Verification items for the finished model (mm, model axes). A direction names the side the tool comes from. Coordinates: 2 decimals unless noted, no trailing zeros. Loops run counter-clockwise (first coordinate to the right, second up) from the corner with the lowest first, then second, coordinate; pieces in that order, holes last. Notation, with made-up numbers: (3.5, -16) - (33.5, -16) arc R26 ccw to (33.5, 21) - close; hole circle Ø11 at (-1.5, 18). An arc over 180 degrees is marked (long way). One line per item, written item: value. Start each with the question number.
(1) Section check C-C (y = -56). Record the boundary of the cut face in (x, z), plus the area to 4 significant figures.
(2) Section check B-B (z = 581). Record the boundary of the cut face in (x, y).
(3) Section check A-A (x = 31). Record the boundary of the cut face in (y, z), plus the area to 3 significant figures.
(4) Gauge pin test, flat ends, axial feed: P1, Ø1, axis at y = -95, z = 428.5, coming from the -X side; P2, Ø0.9, axis at x = 1, z = 397, coming from the +Y side. Record the tip position at first contact, or that the pin passes through.
(5) Draft check along Y on faces 3 (the face through (2.9, -143, 320)), 4 (the face through (25, -149.5, 320)), 5 (the face through (0, -9, 320)), 6 (the face through (26, -152.4, 320)). Enter one of: +Y half, -Y half, draft (parallel to the pull), parting line (faces both ways), or undercut.
(6) Thickness scan on probe 1 along Y at (x, z) = (23.5, 321); probe 2 along X at (y, z) = (-13.5, 350.5); probe 3 along X at (y, z) = (-45, 486.5). Record the ranges inside material, lowest first. Write a range as [from, to].
(7) Set-up check for faces 1 (the face through (50.8, -75, 320)), 2 (the face through (2.9, -9, 320)): record each of +Z, -Z, +X, -X, +Y, -Y from which the full face is reachable in a straight line by a thin tool's end or side.
```python
from build123d import *

# Parameters (mm, degrees)
SALIENTE_EXTRUIR1_DEPTH = 650
REDONDEO1_R             = 2


with BuildPart() as part:
    # Croquis1 → Saliente-Extruir1 (new body)
    with BuildSketch(Plane.XY):
        Polygon((0, 0), (50.8, 0), (50.8, -152.4), (0, -152.4), (0, -137.4), (2.9, -137.4), (2.9, -149.5), (47.9, -149.5), (47.9, -2.9), (2.9, -2.9), (2.9, -15), (0, -15), align=None)
    extrude(amount=SALIENTE_EXTRUIR1_DEPTH)

    # Redondeo1
    redondeo1_edges = [part.edges().sort_by_distance(p)[0] for p in [
        (0, 0, 325),
        (50.8, 0, 325),
        (50.8, -152.4, 325),
        (0, -152.4, 325),
    ]]
    fillet(redondeo1_edges, radius=REDONDEO1_R)


solid = part.part
```
Responses:
1. outline: (47.9, 0) - (50.8, 0) - (50.8, 650) - (47.9, 650) - close
1. area: 1,885 mm²
2. outline: (0, -150.4) arc R2 ccw to (2, -152.4) - (48.8, -152.4) arc R2 ccw to (50.8, -150.4) - (50.8, -2) arc R2 ccw to (48.8, 0) - (2, 0) arc R2 ccw to (0, -2) - (0, -15) - (2.9, -15) - (2.9, -2.9) - (47.9, -2.9) - (47.9, -149.5) - (2.9, -149.5) - (2.9, -137.4) - (0, -137.4) - close
3. outline: (-152.4, 0) - (-149.5, 0) - (-149.5, 650) - (-152.4, 650) - close; (-2.9, 0) - (0, 0) - (0, 650) - (-2.9, 650) - close
3. area: 3,770 mm²
4. P1: stops at x = 47.9
4. P2: stops at y = -0.08
5. face 3: undercut
5. face 4: undercut
5. face 5: draft
5. face 6: -Y half
6. probe 1: y = [-152.4, -149.5], [-2.9, 0]
6. probe 2: x = [0, 2.9], [47.9, 50.8]
6. probe 3: x = [47.9, 50.8]
7. face 1: +Z, -Z, +X, +Y, -Y
7. face 2: +Z, -Z
